Here's how the part is built. I have some questions about the finished solid (model axes, mm). A direction names the side the tool comes from. Coordinates: 2 decimals unless noted, no trailing zeros. Order: outer loops, then holes, each group sorted by start corner. A loop starts at its lowest first (then second) coordinate and runs counter-clockwise, first axis right, second up.
```python
from build123d import *

# Parameters (mm, degrees)
BOSS_EXTRUDE1_DEPTH = 24.13
SKETCH2_W           = 2.54
SKETCH2_H           = 1.27
BOSS_EXTRUDE2_DEPTH = 0.635
CUT_EXTRUDE1_REACH  = 22.373
SKETCH3_W           = 0.984815379
SKETCH3_H           = 0.139763968


with BuildPart() as part:
    # Sketch1 → Boss-Extrude1 (new body)
    with BuildSketch(Plane.XY):
        Polygon((-5.715, 3.175), (-5.715, -3.175), (-4.699, -3.175), (-4.699, -3.429), (-5.969, -3.429), (-5.969, 3.429), (5.969, 3.429), (5.969, -3.429), (4.699, -3.429), (4.699, -3.175), (5.715, -3.175), (5.715, 3.175), align=None)
    extrude(amount=BOSS_EXTRUDE1_DEPTH)

    # Sketch2 → Boss-Extrude2 (add)
    with BuildSketch(Plane(origin=(0, 3.429, 0), x_dir=(1, 0, 0), z_dir=(0, 1, 0))):
        with Locations((0, -4.445)):
            Rectangle(SKETCH2_W, SKETCH2_H)
    extrude(amount=BOSS_EXTRUDE2_DEPTH)

    # Sketch3 → Cut-Extrude1 (cut, up to next)
    with BuildSketch(Plane.XY.offset(5.08), mode=Mode.PRIVATE) as cut_extrude1_sk1:
        with Locations((-0.110929993, 3.498881984)):
            Rectangle(SKETCH3_W, SKETCH3_H)
    cut_extrude1_tool1 = extrude(cut_extrude1_sk1.sketch, amount=-CUT_EXTRUDE1_REACH, mode=Mode.PRIVATE) & part.part
    add(cut_extrude1_tool1.solids().sort_by_distance((-0.11093, 3.498882, 5.08))[0], mode=Mode.SUBTRACT)


solid = part.part
```
Q1. I need wall thicknesses on L1, parallel to X at y = 0.25, z = 16.25 (3 decimals); L2, parallel to Y at x = -3.75, z = 11.5 (3 decimals). Which ranges of each line are inside material? Lowest first, please.
Q2. If we section it at A-A on y = -1.5: Write out the boundary of the cut face in (x, z) (3 decimals), then the cut area to 3 significant figures.
Q3. Will these pins go through, and if not, where does the flat tip stop? pin 1 (1.1 mm diameter, centred on x = 5, z = 13, fed in from +Y); pin 2 (0.5 mm diameter, centred on y = 4, z = 4.5, fed in from +X); pin 3 (0.8 mm diameter, centred on x = 0, z = 4.5, fed in from -Y) (3 decimals).
Q4. If we section it at B-B on z = 4.75: Write out the boundary of the cut face in (x, y) (3 decimals), then the cut area to 3 significant figures.
Q5. We'd pull the mould along X, two halves only. Please class faces 3 (the flat face through (5.715, 0, 12)), 4 (the flat face through (-5.715, 0, 12)), 5 (the flat face through (5.969, 0, 12)), 6 (the flat face through (0, 4.064, 4)): pulls with the +X half, pulls with the -X half, needs draft (parallel to the pull), parting line crosses it, or undercut.
Q6. If we section it at D-D on x = 4: Write out the boundary of the cut face in (y, z) (3 decimals).
Q7. For faces 1 (the flat face through (-5.969, 0, 12)), 2 (the flat face through (-5, -3.175, 12)), which set-ups out of +Z, -Z, +X, -X, +Y, -Y let a thin tool reach every point of the face, with its end or its side?
Q8. If we section it at C-C on z = 8: Write out the boundary of the cut face in (x, y) (3 decimals), then the cut area to 3 significant figures.
Reply:
1. L1: x = -5.969 to -5.715, 5.715 to 5.969
1. L2: y = 3.175 to 3.429
2. outline: (-5.969, 0) - (-5.715, 0) - (-5.715, 24.13) - (-5.969, 24.13) - close; (5.715, 0) - (5.969, 0) - (5.969, 24.13) - (5.715, 24.13) - close
2. area: 12.3 mm2
3. pin 1: stops at y = 3.43
3. pin 2: stops at x = 1.27
3. pin 3: stops at y = 3.175
4. outline: (-5.969, -3.429) - (-4.699, -3.429) - (-4.699, -3.175) - (-5.715, -3.175) - (-5.715, 3.175) - (5.715, 3.175) - (5.715, -3.175) - (4.699, -3.175) - (4.699, -3.429) - (5.969, -3.429) - (5.969, 3.429) - (1.27, 3.429) - (1.27, 4.064) - (-1.27, 4.064) - (-1.27, 3.429) - (-5.969, 3.429) - close; hole (-0.603, 3.429) - (0.381, 3.429) - (0.381, 3.569) - (-0.603, 3.569) - close
4. area: 8.38 mm2
5. face 3: undercut
5. face 4: undercut
5. face 5: pulls with the +X half
5. face 6: needs draft
6. outline: (3.175, 0) - (3.429, 0) - (3.429, 24.13) - (3.175, 24.13) - close
7. face 1: +Z, -Z, -X, +Y, -Y
7. face 2: +Z, -Z
8. outline: (-5.969, -3.429) - (-4.699, -3.429) - (-4.699, -3.175) - (-5.715, -3.175) - (-5.715, 3.175) - (5.715, 3.175) - (5.715, -3.175) - (4.699, -3.175) - (4.699, -3.429) - (5.969, -3.429) - (5.969, 3.429) - (-5.969, 3.429) - close
8. area: 6.90 mm2
